Could you check a few things on this model? Use its own coordinates, in mm. Coordinates: 2 decimals unless noted, no trailing zeros. Order: outer loops, then holes, each group sorted by start corner. A loop starts at its lowest first (then second) coordinate and runs counter-clockwise, first axis right, second up. Notation, with made-up numbers: (64.25, 30.5) - (74.25, 30.5) arc R11 cw to (74.25, 35.5) - close; hole circle Ø1 at (56.5, 14). An arc over 180 degrees is marked (long way). Answer as a JSON object with one key per item and string values. Group by question number.
(1) Imagine slicing it at C-C, the plane z = 2.5. Give the number of separate pieces and of enclosed holes in the cut face, and give its area (3 significant figures).
(2) Will these pins go through, and if not, where does the flat tip stop? P1, Ø1.7, axis at x = 56.35, y = -28.6, coming from the -Z side; P2, Ø1.5, axis at x = 82, z = 1, coming from the -Y side.
(3) Please list where these lines run through material, in increasing order: probe 1 along X at (y, z) = (-39.5, 0.6); probe 2 along X at (y, z) = (-28, 3); probe 3 along Y at (x, z) = (69, 0.35).
(4) Imagine slicing it at B-B, the plane x = 82. Write out the boundary of the cut face in (y, z) (3 decimals).
(5) We'd pull the mould along X, two halves only. Please class faces 1 (the cylindrical face through (75.814, -38.959, 1.61)), 2 (the cylindrical face through (62.605, -38.846, 1.61)), 3 (the flat face through (69, -17.621, 2)), 4 (the cylindrical face through (88.31, -18.12, 1.61)): pulls with the +X half, pulls with the -X half, needs draft (parallel to the pull), parting line crosses it, or undercut.
(6) Imagine slicing it at A-A, the plane y = -26.5. Write out the boundary of the cut face in (x, z) (3 decimals), and give its area (3 significant figures).
(7) Imagine slicing it at D-D, the plane y = -21. Write out the boundary of the cut face in (x, z) (3 decimals), and give its area (3 significant figures).
from build123d import *

# Parameters (mm, degrees)
SKETCH1_R           = 22.38375
BOSS_EXTRUDE1_DEPTH = 3.175
CUT_EXTRUDE1_REACH  = 5.175
SKETCH2_R           = 38.03700281
CUT_EXTRUDE3_REACH  = 5.175
SKETCH4_R           = 1.397
SKETCH4_R_2         = 0.762
BOSS_EXTRUDE2_DEPTH = 3.175
CUT_EXTRUDE4_REACH  = 5.175
SKETCH8_R           = 3.175


with BuildPart() as part:
    # Sketch1 → Boss-Extrude1 (new body)
    with BuildSketch(Plane.XY):
        with Locations((69.054102373, -28.60314574)):
            Circle(SKETCH1_R)
    extrude(amount=BOSS_EXTRUDE1_DEPTH)

    # Sketch2 → Cut-Extrude1 (cut, up to next)
    with BuildSketch(Plane.XY.offset(3.175), mode=Mode.PRIVATE) as cut_extrude1_sk1:
        with Locations((69.054102373, 12.564876285)):
            Circle(SKETCH2_R)
    cut_extrude1_tool1 = extrude(cut_extrude1_sk1.sketch, amount=-CUT_EXTRUDE1_REACH, mode=Mode.PRIVATE) & part.part
    add(cut_extrude1_tool1.solids().sort_by_distance((69.054102, 12.564876, 3.175))[0], mode=Mode.SUBTRACT)

    # Sketch4 → Cut-Extrude3 (cut, up to next)
    with BuildSketch(Plane.XY.offset(3.175), mode=Mode.PRIVATE) as cut_extrude3_sk1:
        with Locations((56.354102373, -28.60314574)):
            Circle(SKETCH4_R)
    cut_extrude3_tool1 = extrude(cut_extrude3_sk1.sketch, amount=-CUT_EXTRUDE3_REACH, mode=Mode.PRIVATE) & part.part
    add(cut_extrude3_tool1.solids().sort_by_distance((56.354102, -28.603146, 3.175))[0], mode=Mode.SUBTRACT)
    # Sketch4 → Cut-Extrude3 (cut, up to next)
    with BuildSketch(Plane.XY.offset(3.175), mode=Mode.PRIVATE) as cut_extrude3_sk2:
        with Locations((81.754102373, -28.60314574)):
            Circle(SKETCH4_R)
    cut_extrude3_tool2 = extrude(cut_extrude3_sk2.sketch, amount=-CUT_EXTRUDE3_REACH, mode=Mode.PRIVATE) & part.part
    add(cut_extrude3_tool2.solids().sort_by_distance((81.754102, -28.603146, 3.175))[0], mode=Mode.SUBTRACT)
    # Sketch4 → Cut-Extrude3 (cut, up to next)
    with BuildSketch(Plane.XY.offset(3.175), mode=Mode.PRIVATE) as cut_extrude3_sk3:
        with Locations((62.704102373, -39.601668368)):
            Circle(SKETCH4_R_2)
    cut_extrude3_tool3 = extrude(cut_extrude3_sk3.sketch, amount=-CUT_EXTRUDE3_REACH, mode=Mode.PRIVATE) & part.part
    add(cut_extrude3_tool3.solids().sort_by_distance((62.704102, -39.601668, 3.175))[0], mode=Mode.SUBTRACT)
    # Sketch4 → Cut-Extrude3 (cut, up to next)
    with BuildSketch(Plane.XY.offset(3.175), mode=Mode.PRIVATE) as cut_extrude3_sk4:
        with Locations((75.404102373, -39.601668368)):
            Circle(SKETCH4_R_2)
    cut_extrude3_tool4 = extrude(cut_extrude3_sk4.sketch, amount=-CUT_EXTRUDE3_REACH, mode=Mode.PRIVATE) & part.part
    add(cut_extrude3_tool4.solids().sort_by_distance((75.404102, -39.601668, 3.175))[0], mode=Mode.SUBTRACT)

    # Sketch7 → Boss-Extrude2 (add)
    with BuildSketch(Plane.XY.offset(3.175)):
        with BuildLine():
            Line((51.503315193, -17.621357289), (86.604889553, -17.621357289))
            ThreePointArc((86.604889553, -17.621357289), (88.334582305, -18.133879499), (89.505846111, -19.505979033))
            ThreePointArc((89.505846111, -19.505979033), (69.054102373, -25.472126525), (48.602358634, -19.505979033))
            ThreePointArc((48.602358634, -19.505979033), (49.77362244, -18.133879499), (51.503315193, -17.621357289))
        make_face()
    extrude(amount=-BOSS_EXTRUDE2_DEPTH)

    # Sketch8 → Cut-Extrude4 (cut, up to next)
    with BuildSketch(Plane.XY.offset(3.175), mode=Mode.PRIVATE) as cut_extrude4_sk1:
        with Locations((69.054102373, -28.60314574)):
            Circle(SKETCH8_R)
    cut_extrude4_tool1 = extrude(cut_extrude4_sk1.sketch, amount=-CUT_EXTRUDE4_REACH, mode=Mode.PRIVATE) & part.part
    add(cut_extrude4_tool1.solids().sort_by_distance((69.054102, -28.603146, 3.175))[0], mode=Mode.SUBTRACT)


solid = part.part
Result set:
{
 "1": {"separate pieces": "1", "enclosed holes": "5", "area": "1,210 mm^2"},
 "2": {"P1": "passes through", "P2": "stops at y = -47.37"},
 "3": {"probe 1": "x = 49.5 to 61.95, 63.46 to 74.65, 76.16 to 88.61", "probe 2": "x = 46.68 to 55.09, 57.61 to 65.94, 72.17 to 80.49, 83.01 to 91.43", "probe 3": "y = -50.99 to -31.78, -25.43 to -17.62"},
 "4": {"outline": "(-46.863, 0) - (-29.978, 0) - (-29.978, 3.175) - (-46.863, 3.175) - close; (-27.228, 0) - (-17.621, 0) - (-17.621, 3.175) - (-27.228, 3.175) - close"},
 "5": {"face 1": "undercut", "face 2": "undercut", "face 3": "needs draft", "face 4": "pulls with the +X half"},
 "6": {"outline": "(46.769, 0) - (66.676, 0) - (66.676, 3.175) - (46.769, 3.175) - close; (71.433, 0) - (91.339, 0) - (91.339, 3.175) - (71.433, 3.175) - close", "area": "126 mm^2"},
 "7": {"outline": "(48.001, 0) - (90.107, 0) - (90.107, 3.175) - (48.001, 3.175) - close", "area": "134 mm^2"}
}
